```python
from build123d import *

# Parameters (mm, degrees)
SKETCH3_W = 0.254
SKETCH3_H = 0.508


with BuildPart() as part:
    # Sketch1 → Revolve1 (revolve)
    with BuildSketch(Plane.XY):
        Polygon((0, 0), (0, 2.3749), (42.0624, 2.3749), (42.0624, 7.21995), (57.912, 7.21995), (57.912, 0), align=None)
    revolve(axis=Axis((57.912, 0, 0), (-1, 0, 0)))

    # Sketch2 → Revolve2 (revolve)
    with BuildSketch(Plane.XY):
        Polygon((-12.7, 0), (-12.7, 1.94056), (-12.22756, 2.413), (0, 2.413), (0, 0), align=None)
    revolve(axis=Axis((0, 0, 0), (-1, 0, 0)))

    # Sketch3 → Cut-Revolve1 (revolve, cut)
    with BuildSketch(Plane.XY):
        with Locations((-0.127, 2.413)):
            Rectangle(SKETCH3_W, SKETCH3_H)
    revolve(axis=Axis((0, 0, 0), (-1, 0, 0)), mode=Mode.SUBTRACT)


solid = part.part
```
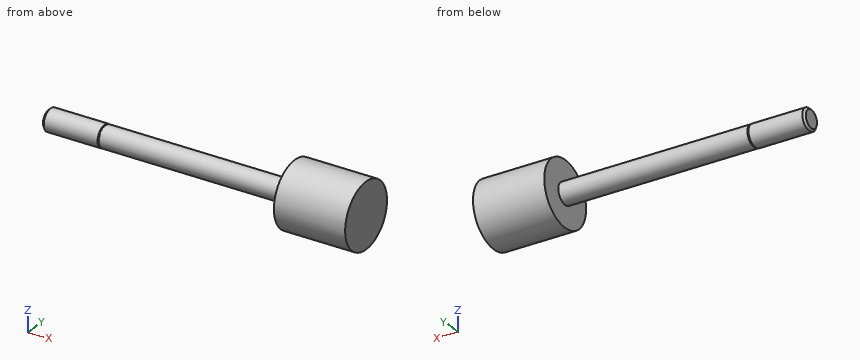
Build history of the part. All positions in model axes, mm. Round coordinates to 2 decimals unless told otherwise and drop trailing zeros. Loops run counter-clockwise (first coordinate to the right, second up) from the corner with the lowest first, then second, coordinate; pieces in that order, holes last. Notation, with made-up numbers: M -2,-14 L 7,-14 A13 cw 7,-8 Z; hole C 23,-10.75 d5. An arc over 180 degrees is marked long. Answer as CSV lines item,"result".
1. Cut at D-D on x = -7.5. Write the cut outline in (y, z).
Resolved:
outline,"C 0,0 d4.83"
2. Flat gauge pins, fed straight in: P1, Ø2, axis at y = 2, z = -4.5, coming from the -X side; P2, Ø6, axis at x = 0, y = -3.5, coming from the +Z side; P3, Ø6, axis at x = 31.5, z = 1.5, coming from the -Y side. Where does each tip first touch, or does it go through?
Resolved:
P1,"stops at x = 42.06"
P2,"stops at z = 2.36"
P3,"stops at y = -2.37"
3. Cut at C-C on x = 47.5. Write the cut outline in (y, z).
Resolved:
outline,"C 0,0 d14.44"
4. Wall check: probe 1 along X at (y, z) = (-3.5, 4.5); probe 2 along Y at (x, z) = (11.5, 0); probe 3 along Y at (x, z) = (24.5, 1.5). Give the ranges that are in metal, low to high. Write a range as [from, to].
Resolved:
probe 1,"x = [42.06, 57.91]"
probe 2,"y = [-2.37, 2.37]"
probe 3,"y = [-1.84, 1.84]"
5. Cut at A-A on z = 0. Write the cut outline in (x, y), then the cut area to 3 significant figures.
Resolved:
outline,"M -12.7,-1.94 L -12.23,-2.41 L -0.25,-2.41 L -0.25,-2.16 L 0,-2.16 L 0,-2.37 L 42.06,-2.37 L 42.06,-7.22 L 57.91,-7.22 L 57.91,7.22 L 42.06,7.22 L 42.06,2.37 L 0,2.37 L 0,2.16 L -0.25,2.16 L -0.25,2.41 L -12.23,2.41 L -12.7,1.94 Z"
area,"490 mm²"
